For this review, use the dimensioned drawing (mm, ordinates from the lowest corner) and the shaded views. A direction names the side the tool comes from. Round coordinates to 2 decimals unless told otherwise and drop trailing zeros. Loops run counter-clockwise (first coordinate to the right, second up) from the corner with the lowest first, then second, coordinate; pieces in that order, holes last. Notation, with made-up numbers: M 32,36.5 L 70,36.5 A22 ccw 70,44.5 Z; hole C 77.25,72 d5. An arc over 180 degrees is marked long. Write item = value, one per line. Start each with the question number.
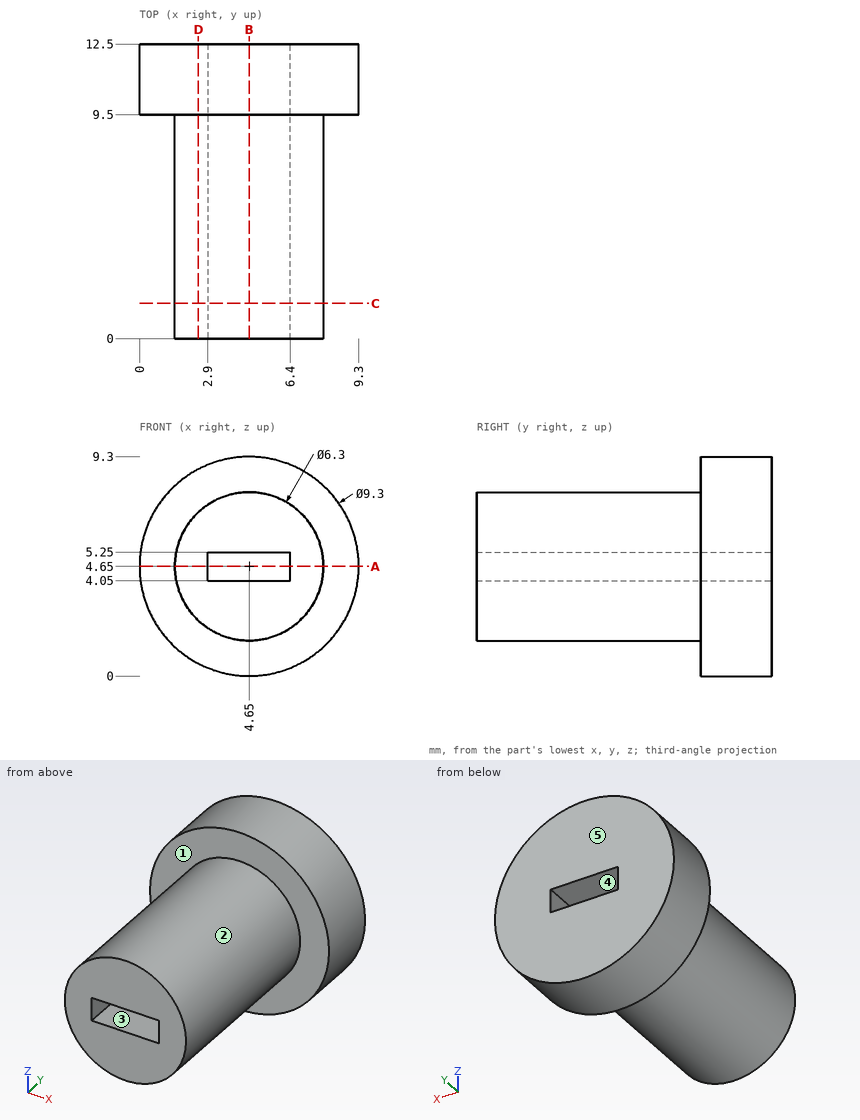
(1) Add section A-A on z = 4.65. Write out the cut boundary in (x, y), and give its area (3 significant figures).
(2) For pin 1 Ø0.6 at (y, z) = (5, 4.5) entering from +X; pin 2 Ø4 at (x, y) = (4, 4.5) entering from +Z; pin 3 Ø3 at (x, y) = (5, 4) entering from -Z, all flat-tipped, find the tip position at first contact; note any pin that passes through.
(3) Wall thickness on L1, parallel to X at y = 8.5, z = 4.5; L2, parallel to Z at x = 3.75, y = 2; L3, parallel to Y at x = 9, z = 4.5: over which ranges is each line inside the solid? List them lowest first.
(4) Add section D-D on x = 2.5. Write out the cut boundary in (y, z).
(5) Tool access review of the marked faces 4 and 5: name each direction out of +Z, -Z, +X, -X, +Y, -Y from which nothing blocks a thin tool from reaching the whole face with its end or side.
(6) Draft analysis for pull direction Z (two halves, no side actions). For the marked faces 1, 2 and 3, state which applies: +Z half, -Z half, draft (parallel to the pull), parting line (faces both ways), or undercut.
(7) Add section B-B on x = 4.65. Write out the cut boundary in (y, z), and give its area (4 significant figures).
(8) Add section C-C on y = 1.5. Write out the cut boundary in (x, z), and give its area (3 significant figures).
Answer sheet:
q1.outline = M 0,9.5 L 1.5,9.5 L 1.5,0 L 2.9,0 L 2.9,12.5 L 0,12.5 Z; M 6.4,0 L 7.8,0 L 7.8,9.5 L 9.3,9.5 L 9.3,12.5 L 6.4,12.5 Z
q1.area = 44.0 mm²
q2.pin_1 = 7.8
q2.pin_2 = 7.8
q2.pin_3 = 1.5
q3.L1 = 1.5 to 2.9, 6.4 to 7.8
q3.L2 = 1.63 to 4.05, 5.25 to 7.67
q3.L3 = 9.5 to 12.5
q4.outline = M 0,2.35 L 9.5,2.35 L 9.5,0.53 L 12.5,0.53 L 12.5,8.77 L 9.5,8.77 L 9.5,6.95 L 0,6.95 Z
q5.face_4 = +Y, -Y
q5.face_5 = +Z, -Z, +X, -X, +Y
q6.face_1 = draft
q6.face_2 = parting line
q6.face_3 = undercut
q7.outline = M 0,1.5 L 9.5,1.5 L 9.5,0 L 12.5,0 L 12.5,4.05 L 0,4.05 Z; M 0,5.25 L 12.5,5.25 L 12.5,9.3 L 9.5,9.3 L 9.5,7.8 L 0,7.8 Z
q7.area = 72.75 mm²
q8.outline = C 4.65,4.65 d6.3; hole M 2.9,4.05 L 6.4,4.05 L 6.4,5.25 L 2.9,5.25 Z
q8.area = 27.0 mm²
